Geometry check sheet. Reference: the model listing, model coordinates, mm. Face numbers are marked on the shaded views. Give positions to 0.01 mm unless a question says otherwise; leave off trailing zeros. Loops run counter-clockwise (first coordinate to the right, second up) from the corner with the lowest first, then second, coordinate; pieces in that order, holes last. Notation, with made-up numbers: (17.25, 19) - (36.25, 19) arc R16 ccw to (36.25, 50) - close; hole circle Ø7 at (56, -24). An arc over 180 degrees is marked (long way). Use a Markdown table: item, result. Add a question column.
1. Cross-section at D-D on x = 16.5. Enter the section's corners in (y, z), and give its area (3 significant figures).
2. Draft check along Z on the marked faces 1, 2 and 3. Enter one of: pulls with the +Z half, pulls with the -Z half, needs draft (parallel to the pull), parting line crosses it, or undercut.
3. Cross-section at C-C on z = 65. Enter the section's corners in (x, y).
4. Material ranges on L1, parallel to X at y = -7.25, z = 72.39; L2, parallel to Z at x = 43, y = 7; L3, parallel to X at y = -9, z = 72, recorded low to high.
5. Cross-section at A-A on z = 79.8. Enter the section's corners in (x, y).
6. Depth check by flat-ended pin: P1, Ø4, axis at x = 13.5, z = 70, coming from the +Y side; P2, Ø1.9, axis at x = 42, y = 8.5, coming from the +Z side; P3, Ø8.5, axis at x = 43, z = 22, coming from the +Y side; P4, Ø1.9, axis at x = -46, y = -8.5, coming from the -Z side. Enter the tip coordinate at first touch or a pass-through.
7. Cross-section at B-B on y = -36.5. Enter the section's corners in (x, z).
from build123d import *

# Parameters (mm, degrees)
SKETCH1_R               = 1.89865
BOSS_EXTRUDE1_DEPTH     = 6.35
SKETCH2_W               = 142.748
SKETCH2_H               = 12.7
BOSS_EXTRUDE2_DEPTH     = 88.9
SKETCH3_W               = 7.62
SKETCH3_H               = 7.62
SKETCH3_R               = 1.69999914
BOSS_EXTRUDE3_DEPTH     = 3.81
CUT_EXTRUDE2_REACH      = 139.396
SKETCH4_R               = 1.69999914
SKETCH4_W               = 81.221287992
SKETCH4_H               = 38.1
SKETCH5_W               = 7.62
SKETCH5_H               = 7.62
SKETCH5_R               = 1.65
BOSS_EXTRUDE4_DEPTH     = 3.81
BOSS_EXTRUDE5_DEPTH     = 6.35
CUT_EXTRUDE3_DEPTH      = 149.43301976
CUT_EXTRUDE3_DEPTH_BACK = 149.43301976
SKETCH9_R               = 1.65
CUT_EXTRUDE4_DEPTH      = 4.365625


with BuildPart() as part:
    # Sketch1 → Boss-Extrude1 (new body)
    with BuildSketch(Plane.XY):
        with BuildLine():
            Line((-71.374, -29.0845), (-71.374, -67.773392633))
            ThreePointArc((-71.374, -67.773392633), (-67.660178189, -71.481332615), (-63.754, -74.986052763))
            Line((-63.754, -74.986052763), (-63.754, -29.0845))
            Line((-63.754, -29.0845), (63.754, -29.0845))
            Line((63.754, -29.0845), (63.754, -74.986052763))
            ThreePointArc((63.754, -74.986052763), (67.660178189, -71.481332615), (71.374, -67.773392633))
            Line((71.374, -67.773392633), (71.374, -29.0845))
            Line((71.374, -29.0845), (71.374, 29.0845))
            Line((71.374, 29.0845), (-71.374, 29.0845))
            Line((-71.374, 29.0845), (-71.374, -29.0845))
        make_face()
        with Locations((-63.754, 21.4645)):
            Circle(SKETCH1_R, mode=Mode.SUBTRACT)
        with Locations((0, 21.4645)):
            Circle(SKETCH1_R, mode=Mode.SUBTRACT)
        with Locations((63.754, 21.4645)):
            Circle(SKETCH1_R, mode=Mode.SUBTRACT)
        with Locations((63.754, -21.4645)):
            Circle(SKETCH1_R, mode=Mode.SUBTRACT)
        with Locations((0, -21.4645)):
            Circle(SKETCH1_R, mode=Mode.SUBTRACT)
        with Locations((-63.754, -21.4645)):
            Circle(SKETCH1_R, mode=Mode.SUBTRACT)
    extrude(amount=BOSS_EXTRUDE1_DEPTH)

    # Sketch2 → Boss-Extrude2 (add)
    with BuildSketch(Plane.XY.offset(6.35)):
        Rectangle(SKETCH2_W, SKETCH2_H)
    extrude(amount=BOSS_EXTRUDE2_DEPTH)

    # Sketch3 → Boss-Extrude3 (add)
    # profile 1 of 4: a face of its own
    with BuildSketch(Plane.XZ.offset(6.35)):
        with Locations((-46.99, 72.39)):
            Rectangle(SKETCH3_W, SKETCH3_H)
        with Locations(Location((-46.99, 72.39, 0), (0, 0, 90))):
            Circle(SKETCH3_R, mode=Mode.SUBTRACT)
    # profile 2 of 4: a face of its own
    with BuildSketch(Plane.XZ.offset(6.35)):
        with Locations((46.99, 72.39)):
            Rectangle(SKETCH3_W, SKETCH3_H)
        with Locations(Location((46.99, 72.39, 0), (0, 0, 90))):
            Circle(SKETCH3_R, mode=Mode.SUBTRACT)
    # profile 3 of 4: a face of its own
    with BuildSketch(Plane.XZ.offset(6.35)):
        with Locations((46.99, 29.21)):
            Rectangle(SKETCH3_W, SKETCH3_H)
        with Locations(Location((46.99, 29.21, 0), (0, 0, 90))):
            Circle(SKETCH3_R, mode=Mode.SUBTRACT)
    # profile 4 of 4: a face of its own
    with BuildSketch(Plane.XZ.offset(6.35)):
        with Locations((-46.99, 29.21)):
            Rectangle(SKETCH3_W, SKETCH3_H)
        with Locations(Location((-46.99, 29.21, 0), (0, 0, 90))):
            Circle(SKETCH3_R, mode=Mode.SUBTRACT)
    extrude(amount=BOSS_EXTRUDE3_DEPTH)

    # Sketch4 → Cut-Extrude2 (cut, up to next)
    with BuildSketch(Plane.XZ.offset(6.35), mode=Mode.PRIVATE) as cut_extrude2_sk1:
        with Locations(Location((-46.99, 29.21, 0), (0, 0, 90))):
            Circle(SKETCH4_R)
    cut_extrude2_tool1 = extrude(cut_extrude2_sk1.sketch, amount=-CUT_EXTRUDE2_REACH, mode=Mode.PRIVATE) & part.part
    # Sketch4 → Cut-Extrude2 (cut, up to next)
    with BuildSketch(Plane.XZ.offset(6.35), mode=Mode.PRIVATE) as cut_extrude2_sk2:
        with Locations(Location((-46.99, 72.39, 0), (0, 0, 90))):
            Circle(SKETCH4_R)
    cut_extrude2_tool2 = extrude(cut_extrude2_sk2.sketch, amount=-CUT_EXTRUDE2_REACH, mode=Mode.PRIVATE) & part.part
    # Sketch4 → Cut-Extrude2 (cut, up to next)
    with BuildSketch(Plane.XZ.offset(6.35), mode=Mode.PRIVATE) as cut_extrude2_sk3:
        with Locations(Location((46.99, 29.21, 0), (0, 0, 90))):
            Circle(SKETCH4_R)
    cut_extrude2_tool3 = extrude(cut_extrude2_sk3.sketch, amount=-CUT_EXTRUDE2_REACH, mode=Mode.PRIVATE) & part.part
    # Sketch4 → Cut-Extrude2 (cut, up to next)
    with BuildSketch(Plane.XZ.offset(6.35), mode=Mode.PRIVATE) as cut_extrude2_sk4:
        with Locations(Location((46.99, 72.39, 0), (0, 0, 90))):
            Circle(SKETCH4_R)
    cut_extrude2_tool4 = extrude(cut_extrude2_sk4.sketch, amount=-CUT_EXTRUDE2_REACH, mode=Mode.PRIVATE) & part.part
    # Sketch4 → Cut-Extrude2 (cut, up to next)
    with BuildSketch(Plane.XZ.offset(6.35), mode=Mode.PRIVATE) as cut_extrude2_sk5:
        with Locations((0, 50.8)):
            Rectangle(SKETCH4_W, SKETCH4_H)
    cut_extrude2_tool5 = extrude(cut_extrude2_sk5.sketch, amount=-CUT_EXTRUDE2_REACH, mode=Mode.PRIVATE) & part.part
    add(cut_extrude2_tool1.solids().sort_by_distance((-46.99, -6.35, 29.21))[0], mode=Mode.SUBTRACT)
    add(cut_extrude2_tool2.solids().sort_by_distance((-46.99, -6.35, 72.39))[0], mode=Mode.SUBTRACT)
    add(cut_extrude2_tool3.solids().sort_by_distance((46.99, -6.35, 29.21))[0], mode=Mode.SUBTRACT)
    add(cut_extrude2_tool4.solids().sort_by_distance((46.99, -6.35, 72.39))[0], mode=Mode.SUBTRACT)
    add(cut_extrude2_tool5.solids().sort_by_distance((0, -6.35, 50.8))[0], mode=Mode.SUBTRACT)

    # Sketch5 → Boss-Extrude4 (add)
    # profile 1 of 4: a face of its own
    with BuildSketch(Plane(origin=(0, 6.35, 0), x_dir=(1, 0, 0), z_dir=(0, 1, 0))):
        with Locations((-43, -21.8)):
            Rectangle(SKETCH5_W, SKETCH5_H)
        with Locations(Location((-43, -21.8, 0), (0, 0, 90))):
            Circle(SKETCH5_R, mode=Mode.SUBTRACT)
    # profile 2 of 4: a face of its own
    with BuildSketch(Plane(origin=(0, 6.35, 0), x_dir=(1, 0, 0), z_dir=(0, 1, 0))):
        with Locations((43, -21.8)):
            Rectangle(SKETCH5_W, SKETCH5_H)
        with Locations(Location((43, -21.8, 0), (0, 0, 90))):
            Circle(SKETCH5_R, mode=Mode.SUBTRACT)
    # profile 3 of 4: a face of its own
    with BuildSketch(Plane(origin=(0, 6.35, 0), x_dir=(1, 0, 0), z_dir=(0, 1, 0))):
        with Locations((43, -79.8)):
            Rectangle(SKETCH5_W, SKETCH5_H)
        with Locations(Location((43, -79.8, 0), (0, 0, 90))):
            Circle(SKETCH5_R, mode=Mode.SUBTRACT)
    # profile 4 of 4: a face of its own
    with BuildSketch(Plane(origin=(0, 6.35, 0), x_dir=(1, 0, 0), z_dir=(0, 1, 0))):
        with Locations((-43, -79.8)):
            Rectangle(SKETCH5_W, SKETCH5_H)
        with Locations(Location((-43, -79.8, 0), (0, 0, 90))):
            Circle(SKETCH5_R, mode=Mode.SUBTRACT)
    extrude(amount=BOSS_EXTRUDE4_DEPTH)

    # Sketch6 → Boss-Extrude5 (add)
    with BuildSketch(Plane.XY.offset(95.25)):
        with BuildLine():
            Line((-71.374, 6.35), (71.374, 6.35))
            Line((71.374, 6.35), (71.374, -6.35))
            Line((71.374, -6.35), (71.374, -67.773392633))
            ThreePointArc((71.374, -67.773392633), (67.660178189, -71.481332615), (63.754, -74.986052763))
            Line((63.754, -74.986052763), (63.754, -29.0845))
            Line((63.754, -29.0845), (-63.754, -29.0845))
            Line((-63.754, -29.0845), (-63.754, -74.986052763))
            ThreePointArc((-63.754, -74.986052763), (-67.660178189, -71.481332615), (-71.374, -67.773392633))
            Line((-71.374, -67.773392633), (-71.374, -6.35))
            Line((-71.374, -6.35), (-71.374, 6.35))
        make_face()
    extrude(amount=BOSS_EXTRUDE5_DEPTH)

    # Sketch9 → Cut-Extrude3 (cut, two sides: drawn at the far end of the back side and taken through both)
    with BuildSketch(Plane(origin=(0, 6.35, 0), x_dir=(1, 0, 0), z_dir=(0, 1, 0)).offset(-CUT_EXTRUDE3_DEPTH_BACK)):
        with Locations(Location((-43, -21.8, 0), (0, 0, 90))):
            Circle(SKETCH9_R)
        with Locations(Location((43, -21.8, 0), (0, 0, 90))):
            Circle(SKETCH9_R)
        with Locations(Location((-43, -79.8, 0), (0, 0, 90))):
            Circle(SKETCH9_R)
        with Locations(Location((43, -79.8, 0), (0, 0, 90))):
            Circle(SKETCH9_R)
    extrude(amount=CUT_EXTRUDE3_DEPTH + CUT_EXTRUDE3_DEPTH_BACK, mode=Mode.SUBTRACT)

    # Sketch10 → Cut-Extrude4 (cut)
    with BuildSketch(Plane.XY.offset(6.35)):
        Polygon((4.16875, 19.057671065), (4.16875, 23.871328935), (0, 26.278157869), (-4.16875, 23.871328935), (-4.16875, 19.057671065), (0, 16.650842131), align=None)
        Polygon((0, -16.650842131), (4.16875, -19.057671065), (4.16875, -23.871328935), (0, -26.278157869), (-4.16875, -23.871328935), (-4.16875, -19.057671065), align=None)
        Polygon((-59.58525, -19.057671065), (-63.754, -16.650842131), (-67.92275, -19.057671065), (-67.92275, -23.871328935), (-63.754, -26.278157869), (-59.58525, -23.871328935), align=None)
        Polygon((-63.754, 16.650842131), (-67.92275, 19.057671065), (-67.92275, 23.871328935), (-63.754, 26.278157869), (-59.58525, 23.871328935), (-59.58525, 19.057671065), align=None)
        Polygon((59.58525, -23.871328935), (59.58525, -19.057671065), (63.754, -16.650842131), (67.92275, -19.057671065), (67.92275, -23.871328935), (63.754, -26.278157869), align=None)
        Polygon((59.58525, 19.057671065), (63.754, 16.650842131), (67.92275, 19.057671065), (67.92275, 23.871328935), (63.754, 26.278157869), (59.58525, 23.871328935), align=None)
    extrude(amount=-CUT_EXTRUDE4_DEPTH, mode=Mode.SUBTRACT)


solid = part.part
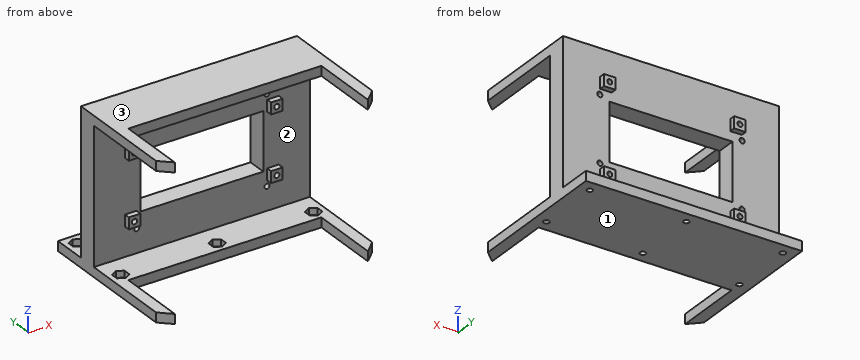
Values found:
| question | item | result |
|---|---|---|
| 1 | outline | (-29.08, 0) - (29.08, 0) - (29.08, 6.35) - (6.35, 6.35) - (6.35, 31.75) - (-6.35, 31.75) - (-6.35, 6.35) - (-29.08, 6.35) - close; (-29.08, 95.25) - (-6.35, 95.25) - (-6.35, 69.85) - (6.35, 69.85) - (6.35, 101.6) - (-29.08, 101.6) - close |
| 1 | area | 1,240 mm2 |
| 2 | face 1 | pulls with the -Z half |
| 2 | face 2 | undercut |
| 2 | face 3 | pulls with the +Z half |
| 3 | outline | (-71.37, -6.35) - (-40.61, -6.35) - (-40.61, 6.35) - (-71.37, 6.35) - close; (40.61, -6.35) - (71.37, -6.35) - (71.37, 6.35) - (40.61, 6.35) - close |
| 4 | L1 | x = -50.8 to -48.69, -45.29 to -43.18, 43.18 to 45.29, 48.69 to 50.8 |
| 4 | L2 | z = 0 to 6.35, 17.99 to 20.15, 23.45 to 25.61, 75.99 to 78.15, 81.45 to 83.61 |
| 4 | L3 | x = -50.8 to -48.64, -45.34 to -43.18, 43.18 to 45.34, 48.64 to 50.8 |
| 5 | outline | (-71.37, -6.35) - (-44.65, -6.35) - (-44.65, 10.16) - (-46.81, 10.16) - (-46.81, 6.35) - (-71.37, 6.35) - close; (-41.35, -6.35) - (41.35, -6.35) - (41.35, 10.16) - (39.19, 10.16) - (39.19, 6.35) - (-39.19, 6.35) - (-39.19, 10.16) - (-41.35, 10.16) - close; (44.65, -6.35) - (71.37, -6.35) - (71.37, 6.35) - (46.81, 6.35) - (46.81, 10.16) - (44.65, 10.16) - close |
| 6 | P1 | stops at y = 6.35 |
| 6 | P2 | stops at z = 83.61 |
| 6 | P3 | stops at y = 10.16 |
| 6 | P4 | stops at z = 0 |
| 7 | outline | (-71.37, 0) - (-63.75, 0) - (-63.75, 6.35) - (-71.37, 6.35) - close; (-71.37, 95.25) - (-63.75, 95.25) - (-63.75, 101.6) - (-71.37, 101.6) - close; (63.75, 0) - (71.37, 0) - (71.37, 6.35) - (63.75, 6.35) - close; (63.75, 95.25) - (71.37, 95.25) - (71.37, 101.6) - (63.75, 101.6) - close |
